```python
from build123d import *

# Parameters (mm, degrees)
BOSS_EXTRUDE5_START                  = -6.35
BOSS_EXTRUDE5_DEPTH                  = 12.7
M3_CLEARANCE_HOLE2_D                 = 3.2
CUT_EXTRUDE2_DEPTH                   = 12.7
BALL_START                           = -6.35
BALL_BALANCER_MASTER_MODEL_OUTLINE_R = 1.6
BALL_BALANCER_MASTER_MODEL_DEPTH     = 12.7


# Read off the part's stored shape, not the designer's step: Ball Balancer Master Model
with BuildPart() as part:
    # Sketch20 → Boss-Extrude5 (new body)
    with BuildSketch(Plane(origin=(0, 24.321911069, 11.341493392), x_dir=(0, -0.4226182617407002, 0.9063077870366497), z_dir=(0, 0.9063077870366496, 0.42261826174070016)).offset(BOSS_EXTRUDE5_START)):
        Polygon((114.700544477, -3.429), (97.238044477, -3.429), (97.238044477, 3.429), (114.700544477, 3.429), (114.700544477, 6.35), (45.701184477, 6.35), (45.701184477, -6.35), (114.700544477, -6.35), align=None)
    extrude(amount=BOSS_EXTRUDE5_DEPTH)

    # M3 Clearance Hole2 (through all)
    with Locations(Plane(origin=(0, 30.076965517, 14.025119355), x_dir=(1, 0, 0), z_dir=(0, 0.9063077870366494, 0.42261826174070066))):
        with Locations((0, -53.551184477)):
            Hole(M3_CLEARANCE_HOLE2_D / 2)

    # Sketch21 → Cut-Extrude2 (cut)
    with BuildSketch(Plane.ZY.offset(6.35)):
        Polygon((66.821464609, 1.208914252), (53.817107939, 7.272945357), (51.884897247, 3.129306154), (64.889253917, -2.93472495), align=None)
    extrude(amount=-CUT_EXTRUDE2_DEPTH, mode=Mode.SUBTRACT)

    # Ball Balancer Master Model outline → Ball Balancer Master Model (cut)
    with BuildSketch(Plane.YZ.offset(BALL_START)):
        with Locations((-21.469007696, 109.540435581)):
            Circle(BALL_BALANCER_MASTER_MODEL_OUTLINE_R)
    extrude(amount=BALL_BALANCER_MASTER_MODEL_DEPTH, mode=Mode.SUBTRACT)


solid = part.part
```
Could you check a few things on this model? Use its own coordinates, in mm. A direction names the side the tool comes from. Coordinates: 2 decimals unless noted, no trailing zeros. Order: outer loops, then holes, each group sorted by start corner. A loop starts at its lowest first (then second) coordinate and runs counter-clockwise, first axis right, second up. Notation, with made-up numbers: M -29,25 L -2,25 A30 ccw -2,60 Z; hole C 2.5,-36 d8. An arc over 180 degrees is marked long. Use a Markdown table: item, result. Add a question column.
Q1. We'd pull the mould along X, two halves only. Please class faces 1 (the flat face through (-0.048, -16.853, 99.432)), 2 (the flat face through (-6.35, -9, 84)), 3 (the flat face through (-3.429, -21, 107)), 4 (the flat face through (4.87, -24.23, 115.26)): pulls with the +X half, pulls with the -X half, needs draft (parallel to the pull), parting line crosses it, or undercut.
Q2. I want a section at D-D on y = -14. List the corners of the cut face in (x, z) for me.
Q3. I want a section at C-C on z = 104.5. List the corners of the cut face in (x, y) for me, then the cut area to 3 significant figures.
Q4. I'm going to push flat-ended pins straight in: pin 1 (1 mm diameter, centred on y = -25, z = 100, fed in from -X); pin 2 (1.5 mm diameter, centred on x = 3, z = 84, fed in from -Y); pin 3 (3 mm diameter, centred on x = -0.5, z = 84.5, fed in from -Y). Where does each tip first touch, or does it pass through?
Q5. I want a section at A-A on x = -2.5. List the corners of the cut face in (y, z) for me.
Q6. Which directions (+Z, -Z, +X, -X, +Y, -Y) give clear straight access to the entire face, cutting with the end or side of a thin tool? Please do faces 5 (the flat face through (3.429, -20, 107)), 6 (the flat face through (-0.09, 4.87, 58.97)), 7 (the cylindrical face through (0.35, -2.81, 59.5)).
Q7. If I drill on L1, parallel to X at y = -24.5, z = 110; L2, parallel to Z at x = 2.5, y = 0.5; L3, parallel to Y at x = -4, z = 56, over which ranges is the centre line in solid material (lowest first)?
Q8. I want a section at B-B on y = -21.5. List the corners of the cut face in (x, z) for me.
Checked values:
| question | item | result |
|---|---|---|
| 1 | face 1 | undercut |
| 1 | face 2 | pulls with the -X half |
| 1 | face 3 | undercut |
| 1 | face 4 | needs draft |
| 2 | outline | M -6.35,78.5 L 6.35,78.5 L 6.35,108.55 L 3.43,108.55 L 3.43,100.76 L -3.43,100.76 L -3.43,108.55 L -6.35,108.55 Z |
| 3 | outline | M -6.35,-26.13 L -3.43,-26.13 L -3.43,-12.11 L -6.35,-12.11 Z; M 3.43,-26.13 L 6.35,-26.13 L 6.35,-12.11 L 3.43,-12.11 Z |
| 3 | area | 81.9 mm² |
| 4 | pin 1 | through |
| 4 | pin 2 | y = -16.92 |
| 4 | pin 3 | y = -17.5 |
| 5 | outline | M -22.53,96.79 L -0.75,50.08 L 3.13,51.88 L -2.93,64.89 L 1.21,66.82 L 7.27,53.82 L 10.76,55.44 L -11.02,102.15 Z |
| 6 | face 5 | +Z, -Y |
| 6 | face 6 | +X, -X |
| 6 | face 7 | none |
| 7 | L1 | -6.35 to -3.43, 3.43 to 6.35 |
| 7 | L2 | 50.66 to 57.52, 66.49 to 77.45 |
| 7 | L3 | -3.51 to 1.21, 6.26 to 10.5 |
| 8 | outline | M -6.35,94.58 L 6.35,94.58 L 6.35,107.94 L 3.43,107.94 L 3.43,97.26 L -3.43,97.26 L -3.43,107.94 L -6.35,107.94 Z; M -6.35,111.14 L -3.43,111.14 L -3.43,116.53 L -6.35,116.53 Z; M 3.43,111.14 L 6.35,111.14 L 6.35,116.53 L 3.43,116.53 Z |
